Read the model definition and answer for the solid it produces. Units are mm, in the model's axes. Give positions to 0.01 mm unless a question says otherwise; leave off trailing zeros. Order: outer loops, then holes, each group sorted by start corner. A loop starts at its lowest first (then second) coordinate and runs counter-clockwise, first axis right, second up. Notation, with made-up numbers: M 6,-32.5 L 34,-32.5 A35 cw 34,6.5 Z; hole C 50.25,46 d9. An arc over 180 degrees is marked long. Write item = value, one per line. Start each with the question number.
from build123d import *

# Parameters (mm, degrees)
EXTRUDE_1_DEPTH     = 3
FILLET_1_R          = 10
SKETCH_2_W          = 14.55
SKETCH_2_H          = 20.5
CUT_EXTRUDE_1_DEPTH = 90.696209507
FILLET_2_R          = 3


with BuildPart() as part:
    # 草图1 → 凸台-拉伸1 (new body)
    with BuildSketch(Plane(origin=(0, 0, 0), x_dir=(1, 0, 0), z_dir=(0, 1, 0))):
        Polygon((10, 0), (10, -3.5), (22, -3.5), (22, 0), (26.95, 0), (26.95, 3.4), (25.55, 3.4), (25.55, 6.8), (26.95, 6.8), (26.95, 10.3), (30.15, 10.3), (30.15, 6.8), (31.55, 6.8), (31.55, 3.4), (30.15, 3.4), (30.15, 0), (35.1, 0), (35.1, -3.5), (47.1, -3.5), (47.1, 0), (51.95, 0), (51.95, 3.4), (50.55, 3.4), (50.55, 6.8), (51.95, 6.8), (51.95, 10.3), (55.15, 10.3), (55.15, 6.8), (56.55, 6.8), (56.55, 3.4), (55.15, 3.4), (55.15, 0), (60.1, 0), (60.1, -3.5), (72.1, -3.5), (72.1, 0), (82.1, 0), (82.1, 32.5), (72.1, 32.5), (72.1, 36), (60.1, 36), (60.1, 32.5), (55.15, 32.5), (55.15, 29.1), (56.55, 29.1), (56.55, 25.7), (55.15, 25.7), (55.15, 22.2), (51.95, 22.2), (51.95, 25.7), (50.55, 25.7), (50.55, 29.1), (51.95, 29.1), (51.95, 32.5), (47.1, 32.5), (47.1, 36), (35.1, 36), (35.1, 32.5), (30.15, 32.5), (30.15, 29.1), (31.55, 29.1), (31.55, 25.7), (30.15, 25.7), (30.15, 22.2), (26.95, 22.2), (26.95, 25.7), (25.55, 25.7), (25.55, 29.1), (26.95, 29.1), (26.95, 32.5), (22, 32.5), (22, 36), (10, 36), (10, 32.5), (0, 32.5), (0, 0), align=None)
    extrude(amount=EXTRUDE_1_DEPTH)

    # 圆角1
    fillet_1_edges = [part.edges().sort_by_distance(p)[0] for p in [
        (0, 1.5, -32.5),
        (82.1, 1.5, -32.5),
        (82.1, 1.5, 0),
        (0, 1.5, 0),
    ]]
    fillet(fillet_1_edges, radius=FILLET_1_R - 0.0001)  # a hair under: the kernel refuses the full size

    # 草图2 → 切除-拉伸1 (cut, through all)
    with BuildSketch(Plane.XZ):
        with Locations((13.275, -16.25)):
            Rectangle(SKETCH_2_W, SKETCH_2_H)
        with Locations((68.925, -16.25)):
            Rectangle(SKETCH_2_W, SKETCH_2_H)
    extrude(amount=-CUT_EXTRUDE_1_DEPTH, mode=Mode.SUBTRACT)

    # 圆角2
    fillet_2_edges = [part.edges().sort_by_distance(p)[0] for p in [
        (6, 1.5, -26.5),
        (6, 1.5, -6),
        (20.55, 1.5, -6),
        (20.55, 1.5, -26.5),
        (61.65, 1.5, -6),
        (76.2, 1.5, -6),
        (76.2, 1.5, -26.5),
        (61.65, 1.5, -26.5),
    ]]
    fillet(fillet_2_edges, radius=FILLET_2_R)


solid = part.part
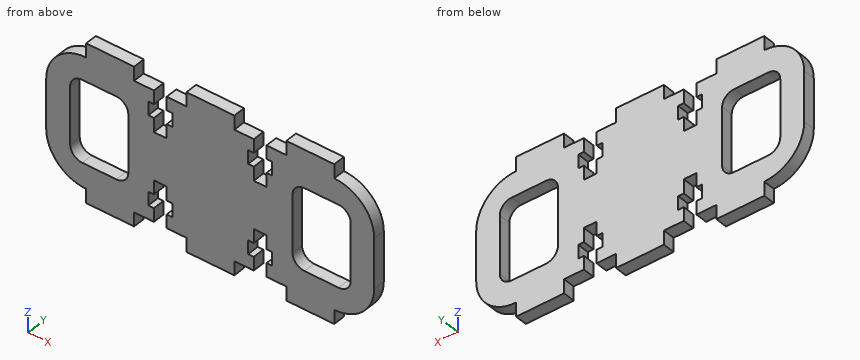
1) Each of these flat-tipped pins is pushed along its axis until it touches: P1, Ø2, axis at x = 16, z = -1.5, coming from the -Y side; P2, Ø1.5, axis at y = 2, z = -1, coming from the -X side; P3, Ø0.9, axis at y = 1.5, z = -30, coming from the -X side; P4, Ø1.5, axis at x = 26, y = 1.5, coming from the -Z side. Where does it stop, or does it pass through?
2) Find section D-D on z = -30. Determine the outline of the cut face in (x, y).
3) Find the intervals of material crossed by probe 1 along X at (y, z) = (2.65, 1); probe 2 along X at (y, z) = (1.5, -22); probe 3 along Z at (x, y) = (64.5, 2.2), in increasing order. Write a range as [from, to].
4) Find section B-B on z = -21. Determine the outline of the cut face in (x, y), plus the area to 3 significant figures.
5) Find section C-C on y = 2.15. Count the separate pieces of the cut face and the enclosed holes in it, plus the area to 3 significant figures.
6) Find section A-A on x = 66.5. Determine the outline of the cut face in (y, z), plus the area to 3 significant figures.
Numbers:
q1.P1 = 0
q1.P2 = 4.35
q1.P3 = 2.91
q1.P4 = -32.5
q2.outline = M 3.39,0 L 26.95,0 L 26.95,3 L 3.39,3 Z; M 30.15,0 L 51.95,0 L 51.95,3 L 30.15,3 Z; M 55.15,0 L 78.71,0 L 78.71,3 L 55.15,3 Z
q3.probe_1 = [10, 22], [35.1, 47.1], [60.1, 72.1]
q3.probe_2 = [0, 6], [20.55, 61.65], [76.2, 82.1]
q3.probe_3 = [-36, -26.5], [-6, 3.5]
q4.outline = M 0,0 L 6,0 L 6,3 L 0,3 Z; M 20.55,0 L 61.65,0 L 61.65,3 L 20.55,3 Z; M 76.2,0 L 82.1,0 L 82.1,3 L 76.2,3 Z
q4.area = 159 mm2
q5.separate_pieces = 1
q5.enclosed_holes = 2
q5.area = 2,080 mm2
q6.outline = M 0,-36 L 3,-36 L 3,-26.5 L 0,-26.5 Z; M 0,-6 L 3,-6 L 3,3.5 L 0,3.5 Z
q6.area = 57.0 mm2
